Can you work these out from the model? Positions are in its coordinate system, mm. Face numbers are marked on the shaded views. A direction names the side the tool comes from. Give positions to 0.01 mm unless a question says otherwise; leave off trailing zeros. Write each loop counter-clockwise with the first axis right and the second up, starting at its lowest first coordinate (ties: lowest second). Pieces come first, ordered by that corner, then holes. Notation, with made-up numbers: (51, 12.5) -> (103, 12.5) arc R16 ccw to (103, 39.5) -> close; hole circle Ø6 at (86.5, -31). An arc over 180 degrees is marked (long way). One line per item, written item: value.
from build123d import *

# Parameters (mm, degrees)
BOSS_EXTRUDE1_DEPTH                            = 4
SKETCH5_R                                      = 4.5
BOSS_EXTRUDE2_DEPTH                            = 2
SKETCH7_W                                      = 6
SKETCH7_H                                      = 14.5
BOSS_EXTRUDE3_DEPTH                            = 15.5
SKETCH13_W                                     = 9
SKETCH13_H                                     = 8
BOSS_EXTRUDE4_DEPTH                            = 15.5
SKETCH6_R                                      = 11.2
CUT_EXTRUDE1_DEPTH                             = 46.469770178
F_2_8_2_8_DIAMETER_HOLE1_D                     = 2.8
CSK_FOR_M3_FLAT_HEAD_MACHINE_SCREW1_AT_2_COUNT = 2
CSK_FOR_M3_FLAT_HEAD_MACHINE_SCREW1_AT_2_PITCH = 25.791089833
CSK_FOR_M3_FLAT_HEAD_MACHINE_SCREW1_AT_3_COUNT = 2
CSK_FOR_M3_FLAT_HEAD_MACHINE_SCREW1_AT_3_PITCH = 25.791089833
CSK_FOR_M3_FLAT_HEAD_MACHINE_SCREW2_AT_2_COUNT = 2
CSK_FOR_M3_FLAT_HEAD_MACHINE_SCREW2_AT_2_PITCH = 25.791089833
CSK_FOR_M3_FLAT_HEAD_MACHINE_SCREW2_AT_3_COUNT = 2
CSK_FOR_M3_FLAT_HEAD_MACHINE_SCREW2_AT_3_PITCH = 25.791089833
FILLET2_R                                      = 1


with BuildPart() as part:
    # Sketch2 → Boss-Extrude1 (new body)
    with BuildSketch(Plane.XY):
        Polygon((-21.5, 35), (-21.5, -35), (-12.5, -35), (-12.5, -21.5), (12.5, -21.5), (12.5, -35), (21.5, -35), (21.5, 35), (12.5, 35), (12.5, 21.5), (-12.5, 21.5), (-12.5, 35), align=None)
    extrude(amount=BOSS_EXTRUDE1_DEPTH)

    # Sketch5 → Boss-Extrude2 (add)
    with BuildSketch(Plane(origin=(0, 0, 0), x_dir=(-1, 0, 0), z_dir=(0, 0, -1))):
        with Locations(Location((-17, 17, 0), (0, 0, 180))):
            Circle(SKETCH5_R)
        with Locations((17, 17)):
            Circle(SKETCH5_R)
        with Locations((17, -17)):
            Circle(SKETCH5_R)
        with Locations(Location((-17, -17, 0), (0, 0, 180))):
            Circle(SKETCH5_R)
    extrude(amount=BOSS_EXTRUDE2_DEPTH)

    # Sketch7 → Boss-Extrude3 (add)
    with BuildSketch(Plane(origin=(0, 0, 0), x_dir=(-1, 0, 0), z_dir=(0, 0, -1))):
        with Locations((0, 14.25)):
            Rectangle(SKETCH7_W, SKETCH7_H)
        with Locations((0, -14.25)):
            Rectangle(SKETCH7_W, SKETCH7_H)
    extrude(amount=BOSS_EXTRUDE3_DEPTH)

    # Sketch13 → Boss-Extrude4 (add)
    with BuildSketch(Plane(origin=(0, 0, 0), x_dir=(-1, 0, 0), z_dir=(0, 0, -1))):
        with Locations((-17, 31)):
            Rectangle(SKETCH13_W, SKETCH13_H)
        with Locations((17, 31)):
            Rectangle(SKETCH13_W, SKETCH13_H)
        with Locations((17, -31)):
            Rectangle(SKETCH13_W, SKETCH13_H)
        with Locations((-17, -31)):
            Rectangle(SKETCH13_W, SKETCH13_H)
    extrude(amount=BOSS_EXTRUDE4_DEPTH)

    # Sketch6 → Cut-Extrude1 (cut, through all)
    with BuildSketch(Plane.XY.offset(4)):
        with Locations((0, 27)):
            Circle(SKETCH6_R)
    cut_extrude1 = extrude(amount=-CUT_EXTRUDE1_DEPTH, mode=Mode.SUBTRACT)

    # Mirror1: Cut-Extrude1 across plane
    add(cut_extrude1.mirror(Plane.ZX), mode=Mode.SUBTRACT)

    # Ø2.8 (2.8) Diameter Hole1 (through all)
    with Locations(Plane.XY.offset(4)):
        with Locations((-17, 17), (17, 17), (17, -17), (-17, -17)):
            Hole(F_2_8_2_8_DIAMETER_HOLE1_D / 2)

    # Sketch9 → CSK for M3 Flat Head Machine Screw1 (revolve, cut)
    with BuildSketch(Plane(origin=(0, 11.604631616, 4), x_dir=(0, -1, 0), z_dir=(1, 0, 0))):
        Polygon((0, 0), (0, 19.5), (1.7, 19.5), (1.7, 3.85), (3.15, 2.4), (3.15, 0), align=None)
    csk_for_m3_flat_head_machine_screw1 = revolve(axis=Axis((0, 11.604631616, 10.35), (0, 0, -1)), mode=Mode.SUBTRACT)

    # CSK for M3 Flat Head Machine Screw1 at 2: CSK for M3 Flat Head Machine Screw1 ×2
    with Locations(*[Vector(0.6591423670083493, 0.7520181779815104, 0) * (i * CSK_FOR_M3_FLAT_HEAD_MACHINE_SCREW1_AT_2_PITCH) for i in range(1, CSK_FOR_M3_FLAT_HEAD_MACHINE_SCREW1_AT_2_COUNT)]):
        add(csk_for_m3_flat_head_machine_screw1, mode=Mode.SUBTRACT)

    # CSK for M3 Flat Head Machine Screw1 at 3: CSK for M3 Flat Head Machine Screw1 ×2
    with Locations(*[Vector(-0.6591423670083494, 0.7520181779815103, 0) * (i * CSK_FOR_M3_FLAT_HEAD_MACHINE_SCREW1_AT_3_PITCH) for i in range(1, CSK_FOR_M3_FLAT_HEAD_MACHINE_SCREW1_AT_3_COUNT)]):
        add(csk_for_m3_flat_head_machine_screw1, mode=Mode.SUBTRACT)

    # Sketch11 → CSK for M3 Flat Head Machine Screw2 (revolve, cut)
    with BuildSketch(Plane(origin=(0, -11.604631616, 4), x_dir=(0, -1, 0), z_dir=(1, 0, 0))):
        Polygon((0, 0), (0, 19.5), (1.7, 19.5), (1.7, 2.85), (3.15, 1.4), (3.15, 0), align=None)
    csk_for_m3_flat_head_machine_screw2 = revolve(axis=Axis((0, -11.604631616, 10.35), (0, 0, -1)), mode=Mode.SUBTRACT)

    # CSK for M3 Flat Head Machine Screw2 at 2: CSK for M3 Flat Head Machine Screw2 ×2
    with Locations(*[Vector(-0.6591423670083494, -0.7520181779815103, 0) * (i * CSK_FOR_M3_FLAT_HEAD_MACHINE_SCREW2_AT_2_PITCH) for i in range(1, CSK_FOR_M3_FLAT_HEAD_MACHINE_SCREW2_AT_2_COUNT)]):
        add(csk_for_m3_flat_head_machine_screw2, mode=Mode.SUBTRACT)

    # CSK for M3 Flat Head Machine Screw2 at 3: CSK for M3 Flat Head Machine Screw2 ×2
    with Locations(*[Vector(0.6591423670083493, -0.7520181779815104, 0) * (i * CSK_FOR_M3_FLAT_HEAD_MACHINE_SCREW2_AT_3_PITCH) for i in range(1, CSK_FOR_M3_FLAT_HEAD_MACHINE_SCREW2_AT_3_COUNT)]):
        add(csk_for_m3_flat_head_machine_screw2, mode=Mode.SUBTRACT)

    # Fillet2
    fillet2_edges = [part.edges().sort_by_distance(p)[0] for p in [
        (9.756536271, 21.5, 2),
        (-9.756536271, 21.5, 2),
        (9.756536271, -21.5, 2),
        (-9.756536271, -21.5, 2),
        (-12.5, 35, -5.75),
        (-12.5, 21.5, 2),
        (12.5, 21.5, 2),
        (12.5, 35, -5.75),
        (21.5, 35, -5.75),
        (21.5, -35, -5.75),
        (12.5, -35, -5.75),
        (12.5, -21.5, 2),
        (-12.5, -21.5, 2),
        (-12.5, -35, -5.75),
        (-21.5, -35, -5.75),
        (-21.5, 35, -5.75),
        (3, 7, -7.75),
        (-3, 7, -7.75),
        (-3, -7, -7.75),
        (3, -7, -7.75),
    ]]
    fillet(fillet2_edges, radius=FILLET2_R)


solid = part.part
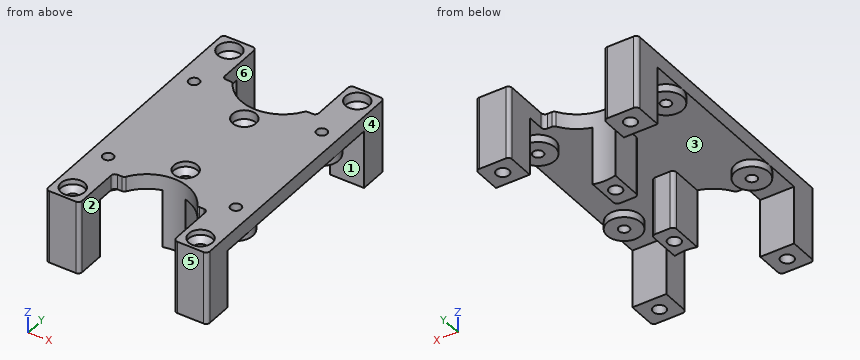
1) Will these pins go through, and if not, where does the flat tip stop? pin 1 (8 mm diameter, centred on y = 18.5, z = -7, fed in from +X); pin 2 (1 mm diameter, centred on x = -6, z = 0.5, fed in from -Y); pin 3 (7 mm diameter, centred on x = 16, y = -15, fed in from -Z).
Answer list:
pin 1: stops at x = 3
pin 2: stops at y = -17.88
pin 3: stops at z = -2
2) For the marked faces 1, 2 and 3, which set-ups out of +Z, -Z, +X, -X, +Y, -Y let a thin tool reach every point of the face, with its end or its side?
Answer list:
face 1: -Z, +X, -X
face 2: +Z, -Z, -Y
face 3: -Z
3) If we section it at B-B (z = -4): State how many separate pieces and enclosed holes the cut face has, and give its area (3 significant figures).
Answer list:
separate pieces: 6
enclosed holes: 6
area: 338 mm^2
4) If we section it at A-A (y = 23.5): Write out the boundary of the cut face in (x, z), and give its area (3 significant figures).
Answer list:
outline: (-21.5, 0) -> (-12.5, 0) -> (-12.5, 4) -> (-21.5, 4) -> close; (12.5, 0) -> (21.5, 0) -> (21.5, 4) -> (12.5, 4) -> close
area: 72.0 mm^2
5) If we section it at D-D (y = -19.5): Write out the boundary of the cut face in (x, z).
Answer list:
outline: (-21.5, 0) -> (-20.74, 0) -> (-20.74, -2) -> (-13.26, -2) -> (-13.26, 0) -> (-8.32, 0) -> (-8.32, 4) -> (-21.5, 4) -> close; (8.32, 0) -> (13.26, 0) -> (13.26, -2) -> (20.74, -2) -> (20.74, 0) -> (21.5, 0) -> (21.5, 4) -> (8.32, 4) -> close
6) We'd pull the mould along X, two halves only. Please class the marked faces 4, 5 and 6: released by +X, released by -X, zero draft, split by the parting line, or undercut.
Answer list:
face 4: released by +X
face 5: zero draft
face 6: undercut
7) I need wall thicknesses on L1, parallel to X at y = -31, z = 3.65; L2, parallel to Y at x = 0, z = -8.75; L3, parallel to Y at x = 19, z = -12.25. Which ranges of each line are inside material? Lowest first, please.
Answer list:
L1: x = -21.5 to -20.15, -13.85 to -12.5, 12.5 to 13.85, 20.15 to 21.5
L2: y = -15.8 to -13.3, -9.9 to -7, 7 to 9.9, 13.3 to 15.8
L3: y = -35 to -27, 27 to 35
